Design review of the part built by this model. Coordinates are the model's own, in mm. Face numbers are marked on the shaded views. A direction names the side the tool comes from. Give positions to 0.01 mm unless a question says otherwise; leave off trailing zeros. Write each loop counter-clockwise with the first axis right and the second up, starting at its lowest first coordinate (ties: lowest second). Pieces come first, ordered by that corner, then holes. Notation, with made-up numbers: (86, -29) -> (143, -29) arc R21 ccw to (143, -1) -> close; hole circle Ø4 at (19, 16). An arc over 180 degrees is marked (long way). Use CSV: the item, a comma, the result in double quotes.
Autodesk Inventor part; units mm, degrees
ref_plane "YZ Plane" through (0, 0, 0) normal (1, 0, 0) x (0, 1, 0)
ref_plane "XZ Plane" through (0, 0, 0) normal (0, 1, 0) x (-1, 0, 0)
ref_plane "XY Plane" through (0, 0, 0) normal (0, 0, 1) x (1, 0, 0)
sketch "Sketch1" plane through (0, 0, 0) normal (0, 1, 0) x (-1, 0, 0)
  arc A0 (0, -5) -> (0, 5) centre (0, 0) ccw
  line L0 (0, 5) -> (0, -5)
  dimension "d0" = 10
extrude "Extrusion1" add sketch "Sketch1" along normal blind 10
sketch "Sketch2" plane through (0, 0, 0) normal (1, 0, 0) x (0, 1, 0)
  line L0 (8.0172, -4.5) -> (8.0172, 4.5)
  line L1 (8.0172, 4.5) -> (2.5172, 4.5)
  line L2 (2.5172, -4.5) -> (0.0172, -2)
  line L3 (2.5172, 4.5) -> (0.0172, 2)
  line L4 (0.0172, -2) -> (0.0172, 2)
  line L5 (8.0172, -4.5) -> (2.5172, -4.5)
  point P0 (0, 0)
  dimension "d3" = 9
  dimension "d4" = 8
sketch "Sketch3" plane through (0, 0, 0) normal (1, 0, 0) x (0, 1, 0)
  line L0 (0, 2) -> (3, 5)
  arc A0 (3, 5) -> (0, 2) centre (1, 4) ccw
  line L1 (0, -2) -> (4, -6)
  arc A1 (0, -2) -> (4, -6) centre (1.75, -4.25) ccw
  line L2 (8.0325, 5) -> (11, 5)
  line L3 (11, 5) -> (11, -6)
  line L4 (11, -6) -> (8.0325, -6)
  line L5 (8.0325, -6) -> (8.0325, 5)
  line L6 (2.4911, 4.4911) -> (5, 7)
  line L7 (2.4911, 4.4911) -> (8.0325, 4.4911)
  arc A2 (8.0325, 4.4911) -> (5, 7) centre (7, 6.3303) ccw
  line L8 (2.4911, -4.4911) -> (8.5706, -4.4911)
  arc A3 (2.4911, -4.4911) -> (8.5706, -4.4911) centre (5.5309, -7.5041) ccw
  point P0 (0, 0)
extrude "Extrusion2" cut sketch "Sketch3" against normal through all
sketch "Sketch4" plane through (0, 0, 0) normal (0, 1, 0) x (-1, 0, 0)
  arc A0 (1.0726, -4.4911) -> (1.0726, 4.4911) centre (-1.125, 0) ccw
  arc A1 (1.0726, 4.4911) -> (1.0726, -4.4911) centre (-0.4517, 0) ccw
  point P0 (0, 0)
  point P1 (2.1976, -4.4911)
  point P2 (2.1976, 4.4911)
  dimension "d9" = 1.125
  dimension "d10" = 1.125
extrude "Extrusion3" cut sketch "Sketch4" along normal through all both and the other way through all
sketch "Sketch5" plane through (0, 0, 0) normal (1, 0, 0) x (0, 1, 0)
  line L0 (1.6, -1.2445) -> (1.6, 1.1555)
  line L1 (6.4325, 2.6911) -> (3.1125, 2.6911)
  line L2 (6.4325, -2.6911) -> (6.4325, 2.6911)
  line L3 (6.4325, -2.6911) -> (3.1125, -2.6911)
  line L4 (0, 2) -> (0, -2)
  line L5 (8.0325, 4.4911) -> (8.0325, -4.4911)
  line L6 (0, 2) -> (2.4911, 4.4911)
  line L7 (2.4911, 4.4911) -> (8.0325, 4.4911)
  line L8 (8.0325, 4.4911) -> (8.0325, -4.4911)
  line L9 (8.0325, -4.4911) -> (2.4911, -4.4911)
  line L10 (2.4911, -4.4911) -> (0, -2)
  line L11 (0, 2) -> (0, -2)
  line L12 (1.6, 1.1555) -> (3.1125, 2.6911)
  line L13 (1.6, -1.2445) -> (3.1125, -2.6911)
  line L14 (1.6, 4.6579) -> (1.6, -5.3823)
  arc A0 (1.6, 4.6579) -> (1.6, -5.3823) centre (3.2437, -0.3622) ccw
  line L15 (1.6, 1.1555) -> (5.4757, 5.0906)
  line L16 (1.6, 1.1555) -> (1.6, 7.5999)
  arc A1 (5.4757, 5.0906) -> (1.6, 7.5999) centre (3.8837, 6.8794) ccw
  line L17 (3.1125, 2.6911) -> (12.4034, 2.6911)
  line L18 (3.1125, 2.6911) -> (8.5318, 8.1936)
  arc A2 (12.4034, 2.6911) -> (8.5318, 8.1936) centre (8.3272, 3.9364) ccw
  line L19 (6.4325, 2.6911) -> (13.6333, 2.6911)
  line L20 (6.4325, 2.6911) -> (6.4325, -9.3636)
  arc A3 (6.4325, -9.3636) -> (13.6333, 2.6911) centre (6.37, -1.1482) ccw
  line L21 (6.4325, -2.6911) -> (6.4325, -11.5775)
  line L22 (6.4325, -2.6911) -> (3.1125, -2.6911)
  line L23 (3.1125, -2.6911) -> (3.2437, -12.8567)
  arc A4 (3.2437, -12.8567) -> (6.4325, -9.3636) centre (5.6123, -11.8169) ccw
  line L24 (1.6, -1.2445) -> (1.6, -8.2222)
  line L25 (1.6, -1.2445) -> (3.1125, -2.6911)
  line L26 (3.1125, -2.6911) -> (3.1946, -9.0574)
  arc A5 (1.6, -8.2222) -> (3.1946, -9.0574) centre (2.6381, -8.1801) ccw
  point P0 (0, 0)
  dimension "d16" = 1.6
  dimension "d18" = 1.6
  dimension "d21" = 1.8
  dimension "d23" = 1.8
  dimension "d24" = 2.4
  dimension "d26" = 3.32
  dimension "d27" = 3.32
extrude "Extrusion4" cut sketch "Sketch5" against normal through all contours L14 L10 L4 L6 L0 | L13 L23 L9 L10 L14 | L14 L6 L7 L15 L12 | L3 L20 L9 L23 | L14 A0 L6 L4 L10 | L10 L9 L23 A5 L24 L14 | L15 L7 L5 L17 L1 | L14 L16 A1 L15 L7 L6 | L2 L17 L5 L9 L20 | L9 L20 A4 L23 | L15 L18 A2 L17 L5 L7 | L9 L5 L17 L19 A3 L20
sketch "Sketch6" plane through (0, 0, 0) normal (1, 0, 0) x (0, 1, 0)
  circle A0 centre (4, 0) radius 2.5
  line L0 (1.6, -1.2445) -> (1.6, 1.1555)
  point P0 (0, 0)
  dimension "d31" = 5
  dimension "d32" = 2.4
extrude "Extrusion5" add sketch "Sketch6" against normal blind 15
sketch "Sketch7" plane through (0, 0, 0) normal (0, 1, 0) x (-1, 0, 0)
  arc A0 (3.089, -2.6911) -> (3.7176, -1.2445) centre (-1.125, 0) ccw
  arc A1 (3.7397, 1.1555) -> (3.089, 2.6911) centre (-1.125, 0) ccw
  arc A2 (3.7176, -1.2445) -> (3.7397, 1.1555) centre (-1.125, 0) ccw
  arc A3 (3.089, 2.6911) -> (3.089, -2.6911) centre (1.3425, 0) ccw
  point P0 (0, 0)
extrude "Extrusion6" cut sketch "Sketch7" along normal through all
sketch "Sketch8" plane through (-15, 4, 0) normal (-1, 0, 0) x (0, 0, 1)
  circle A0 centre (0, 0) radius 0.5375
  point P0 (0, -4)
  dimension "d37" = 1.075
extrude "Extrusion7" cut sketch "Sketch8" against normal blind 7
sketch "Sketch9" plane through (0, 0, 0) normal (0, 1, 0) x (-1, 0, 0)
  line L0 (6, 3) -> (2, 3)
  line L1 (2, 3) -> (2, -3)
  line L2 (2, -3) -> (6, -3)
  line L3 (6, -3) -> (6, 3)
  point P0 (0, 0)
extrude "Extrusion8" cut sketch "Sketch9" along normal through all both and the other way through all
sketch "Sketch10" plane through (-15, 4, 0) normal (-1, 0, 0) x (0, 0, 1)
  circle A0 centre (0, 0) radius 1
  circle A1 centre (0, 0) radius 3.1623
  point P0 (0, -4)
extrude "Extrusion9" cut sketch "Sketch10" against normal blind 8
properties part number "flat_cranial_window_stabilizer_FAT_May1519"
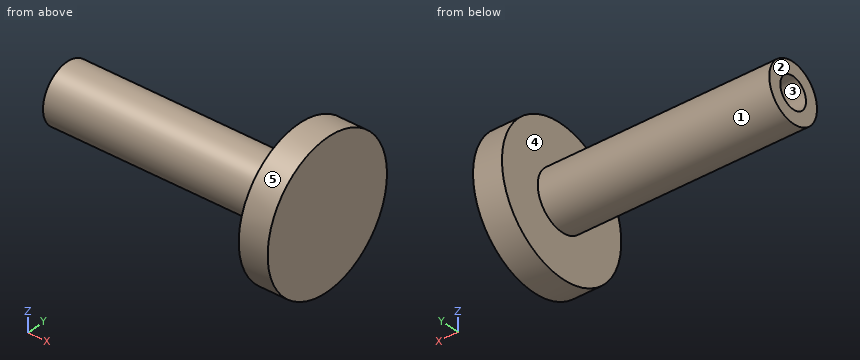
(1) Tool access review of the marked faces 4 and 5: name each direction out of +Z, -Z, +X, -X, +Y, -Y from which nothing blocks a thin tool from reaching the whole face with its end or side.
Established:
face 4,"-X"
face 5,"+X, -X"
(2) Mouldability with a two-part tool opening along Z and no side actions: class the marked faces 1, 2 and 3 as +Z half, -Z half, draft (parallel to the pull), parting line (faces both ways), or undercut.
Established:
face 1,"parting line"
face 2,"draft"
face 3,"undercut"
(3) Take a section at C-C (x = -7.25). Write out the cut boundary in (y, z), then the cut area to 3 significant figures.
Established:
outline,"circle Ø2 at (4, 0)"
area,"3.14 mm2"
(4) For line 1 along Y through (x, z) = (-10.5, 0); line 2 along X through (y, z) = (3.45, -1); line 3 along X through (y, z) = (3.75, 0.05), list the stretches that pass through material, from the lowest coordinate up. Write a range as [from, to].
Established:
line 1,"y = [3, 3.46], [4.54, 5]"
line 2,"x = [-7, -6]"
line 3,"x = [-8, -6]"
(5) Take a section at D-D (x = -12.25). Write out the cut boundary in (y, z) (1 decimal), then the cut area to 3 significant figures.
Established:
outline,"circle Ø2 at (4, 0); hole circle Ø1.1 at (4, 0)"
area,"2.23 mm2"
(6) Take a section at A-A (z = 0). Write out the cut boundary in (x, y), then the cut area to 3 significant figures.
Established:
outline,"(-15, 3) -> (-7, 3) -> (-7, 1.5) -> (-6, 1.5) -> (-6, 6.5) -> (-7, 6.5) -> (-7, 5) -> (-15, 5) -> (-15, 4.54) -> (-8, 4.54) -> (-8, 3.46) -> (-15, 3.46) -> close"
area,"13.5 mm2"
(7) Clearance check with flat-ended pins moving along their axes: pin 1 (1.5 mm diameter, centred on x = -8.5, z = 0, fed in from +Y); pin 2 (1.5 mm diameter, centred on x = -11.5, y = 3, fed in from +Z); pin 3 (0.9 mm diameter, centred on y = 4, z = 0, fed in from -X). State where each tip first meets the part, or that it passes through.
Established:
pin 1,"stops at y = 5"
pin 2,"stops at z = 0.97"
pin 3,"stops at x = -8"
(8) Take a section at B-B (y = 4). Write out the cut boundary in (x, z).
Established:
outline,"(-15, -1) -> (-7, -1) -> (-7, -2.5) -> (-6, -2.5) -> (-6, 2.5) -> (-7, 2.5) -> (-7, 1) -> (-15, 1) -> (-15, 0.54) -> (-8, 0.54) -> (-8, -0.54) -> (-15, -0.54) -> close"
